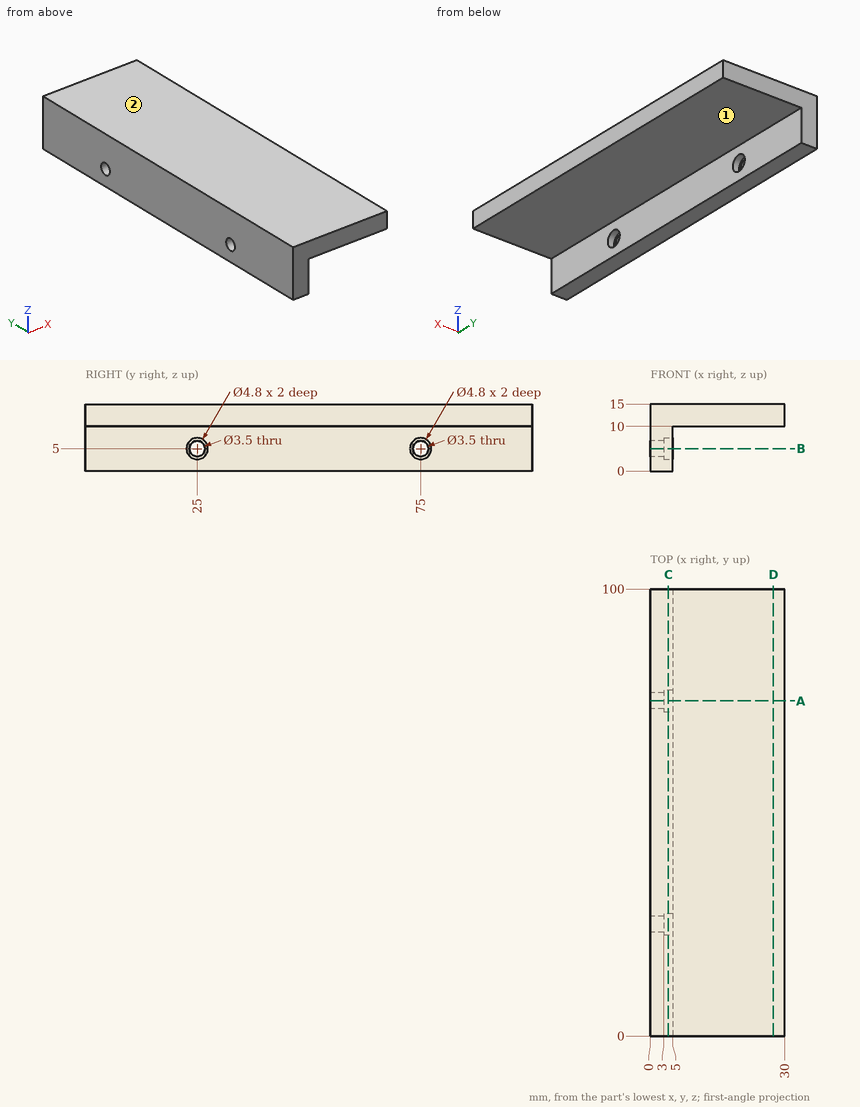
Design review of the part shown in the three views and the two pictorial views. Dimensions are in mm from the part's minimum x, y and z. A direction names the side the tool comes from. Give positions to 0.01 mm unless a question says otherwise; leave off trailing zeros. Loops run counter-clockwise (first coordinate to the right, second up) from the corner with the lowest first, then second, coordinate; pieces in that order, holes last. Notation, with made-up numbers: M 80.5,76 L 105.5,76 A18 cw 105.5,97 Z; hole C 10.5,32.5 d9. An arc over 180 degrees is marked long. Write item = value, one per line.
Q1. For the marked faces 1 and 2, list the 3-axis set-ups (+Z, -Z, +X, -X, +Y, -Y) from which the entire face can be reached by the end or side of a thin tool; tool diameter is ignored.
Output values:
face_1 = -Z, +X, +Y, -Y
face_2 = +Z, +X, -X, +Y, -Y
Q2. We need section A-A (y = 75). Give the boundary of the cut face in (x, z), plus the area to 3 significant figures.
Output values:
outline = M 0,0 L 5,0 L 5,2.6 L 3,2.6 L 3,3.25 L 0,3.25 Z; M 0,6.75 L 3,6.75 L 3,7.4 L 5,7.4 L 5,10 L 30,10 L 30,15 L 0,15 Z
area = 180 mm^2
Q3. Insertion check: pin 1 (7.5 mm diameter, centred on y = 75, z = 5, fed in from +X); pin 2 (3 mm diameter, centred on y = 25, z = 5, fed in from +X); pin 3 (7.5 mm diameter, centred on x = 13.5, y = 64, fed in from -Z); pin 4 (1.4 mm diameter, centred on y = 74, z = 4.5, fed in from +X). Each pin has a flat end and moves straight along its axis. Give the tip position at first contact, or say it passes through.
Output values:
pin_1 = 5
pin_2 = through
pin_3 = 10
pin_4 = 3
Q4. We need section C-C (x = 4). Give the boundary of the cut face in (y, z).
Output values:
outline = M 0,0 L 100,0 L 100,15 L 0,15 Z; hole C 25,5 d4.8; hole C 75,5 d4.8
Q5. We need section B-B (z = 5). Give the boundary of the cut face in (x, y), plus the area to 3 significant figures.
Output values:
outline = M 0,0 L 5,0 L 5,22.6 L 3,22.6 L 3,23.25 L 0,23.25 Z; M 0,26.75 L 3,26.75 L 3,27.4 L 5,27.4 L 5,72.6 L 3,72.6 L 3,73.25 L 0,73.25 Z; M 0,76.75 L 3,76.75 L 3,77.4 L 5,77.4 L 5,100 L 0,100 Z
area = 460 mm^2
Q6. We need section D-D (x = 27.5). Give the boundary of the cut face in (y, z), plus the area to 3 significant figures.
Output values:
outline = M 0,10 L 100,10 L 100,15 L 0,15 Z
area = 500 mm^2
Q7. To check wall thickness, follow line 1 (Z direction, x = 2.15, y = 25); line 2 (Z direction, x = 4.55, y = 25); line 3 (Z direction, x = 9.5, y = 21.5). State the ranges of each line that lie inside material, in increasing order. Write a range as [from, to].
Output values:
line_1 = [0, 3.25], [6.75, 15]
line_2 = [0, 2.6], [7.4, 15]
line_3 = [10, 15]
